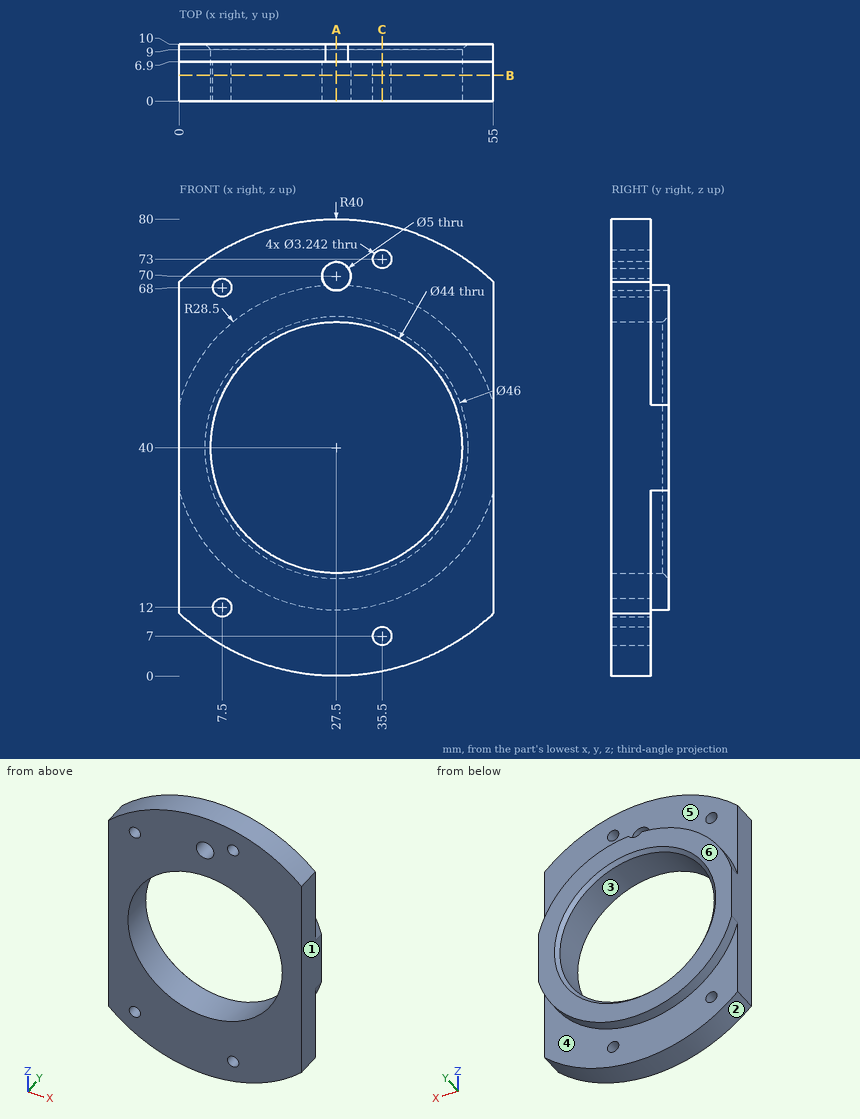
The figure shows three views and two pictorial views of one solid part (mm, origin at its lowest corner). Answer the questions. A direction names the side the tool comes from. Give positions to 0.01 mm unless a question says otherwise; leave off trailing zeros. Loops run counter-clockwise (first coordinate to the right, second up) from the corner with the lowest first, then second, coordinate; pieces in that order, holes last. Notation, with made-up numbers: (60, 16) - (65, 16) arc R19 ccw to (65, 30) - close; hole circle Ø7 at (39, 36.25). An arc over 180 degrees is marked (long way). Use one line per item in the form item = value.
1. Section A-A on x = 27.5 is taken. Give the vertices of the cut face in (y, z).
Calculated:
outline = (0, 0) - (6.9, 0) - (6.9, 11.5) - (10, 11.5) - (10, 17) - (9, 18) - (0, 18) - close; (0, 62) - (9, 62) - (10, 63) - (10, 67.5) - (0, 67.5) - close; (0, 72.5) - (6.9, 72.5) - (6.9, 80) - (0, 80) - close
2. The mould has two halves that part along X. Classify the marked faces 1, 2 and 3: pulls with the +X half, pulls with the -X half, needs draft (parallel to the pull), parting line crosses it, or undercut.
Calculated:
face_1 = pulls with the +X half
face_2 = parting line crosses it
face_3 = undercut
3. Section B-B on y = 4.5 is taken. Give the vertices of the cut face in (x, z), then the cut area to 3 significant figures.
Calculated:
outline = (0, 10.95) arc R40 ccw to (55, 10.95) - (55, 69.05) arc R40 ccw to (0, 69.05) - close; hole circle Ø44 at (27.5, 40); hole circle Ø3.24 at (7.5, 12); hole circle Ø3.24 at (7.5, 68); hole circle Ø5 at (27.5, 70); hole circle Ø3.24 at (35.5, 7); hole circle Ø3.24 at (35.5, 73)
area = 2,450 mm^2
4. Which of the six approach directions +Z, -Z, +X, -X, +Y, -Y give full straight-line access (tool end or side, diameter ignored) to the marked faces 4, 5 and 6?
Calculated:
face_4 = -Z, +Y
face_5 = +Z, +Y
face_6 = +Z, -Z, +X, -X, +Y
5. Section C-C on x = 35.5 is taken. Count the separate pieces of the cut face and the enclosed holes in it, then the cut area to 3 significant figures.
Calculated:
separate_pieces = 4
enclosed_holes = 0
area = 255 mm^2
6. Given pin 1 Ø2 at (y, z) = (8, 8.5) entering from +X; pin 2 Ø2 at (x, z) = (11.5, 68.5) entering from +Y; pin 3 Ø10 at (x, z) = (13.5, 30) entering from +Y, each flat-ended and moving along its own axis, determine where each tip first touches the part or whether it passes through.
Calculated:
pin_1 = through
pin_2 = 6.9
pin_3 = 9.2
7. Find the intervals of material crossed by line 1 along Z through (x, y) = (27.5, 7.25); line 2 along Z through (x, y) = (29, 4); line 3 along Z through (x, y) = (36, 1), in increasing order. Write a range as [from, to].
Calculated:
line_1 = [11.5, 18], [62, 67.5]
line_2 = [0.03, 18.05], [61.95, 68], [72, 79.97]
line_3 = [0.91, 5.46], [8.54, 19.71], [60.29, 71.46], [74.54, 79.09]
